For this review, take the finished solid that the model builds, in its own axes (mm). Face numbers are marked on the shaded views. A direction names the side the tool comes from. Give positions to 0.01 mm unless a question says otherwise; leave off trailing zeros. Order: outer loops, then holes, each group sorted by start corner. A loop starts at its lowest first (then second) coordinate and runs counter-clockwise, first axis right, second up. Notation, with made-up numbers: (-7.75, 21.5) -> (47.25, 21.5) arc R27 ccw to (47.25, 42.5) -> close; hole circle Ø5 at (27, 38.5). An arc over 180 degrees is marked (long way). One line per item, written item: value. Start each with the question number.
from build123d import *

# Parameters (mm, degrees)
PAD_DEPTH        = 8
SKETCH001_W      = 60
SKETCH001_H      = 5
PAD001_DEPTH     = 240
POCKET_DEPTH     = 5.001
POCKET001_DEPTH  = 5.001
PAD002_DEPTH     = 8
HOLE_D           = 4.4
HOLE_CSINK_D     = 8
HOLE_CSINK_ANGLE = 90


with BuildPart() as part:
    # Sketch → Pad (new body)
    with BuildSketch(Plane.XZ):
        with BuildLine():
            Line((-30, 0), (30, 0))
            Line((30, 0), (30, -30))
            Line((30, -30), (20.25, -30))
            Line((20.25, -22.145781), (20.25, -30))
            ThreePointArc((20.25, -22.145781), (14, -10.5), (7.75, -22.145781))
            Line((7.75, -22.145781), (7.75, -30))
            Line((7.75, -30), (-7.75, -30))
            Line((-7.75, -22.145781), (-7.75, -30))
            ThreePointArc((-7.75, -22.145781), (-14, -10.5), (-20.25, -22.145781))
            Line((-20.25, -22.145781), (-20.25, -30))
            Line((-20.25, -30), (-30, -30))
            Line((-30, -30), (-30, 0))
        make_face()
    extrude(amount=PAD_DEPTH)

    # Sketch001 (on Face14 of Pad) → Pad001 (join)
    with BuildSketch(Plane.XZ.offset(8)):
        with Locations((0, -2.5)):
            Rectangle(SKETCH001_W, SKETCH001_H)
    extrude(amount=PAD001_DEPTH)

    # Sketch002 (on Face15 of Pad001) → Pocket (cut, through all)
    with BuildSketch(Plane(origin=(0, 0, -5), x_dir=(1, 0, 0), z_dir=(0, 0, -1))):
        Polygon((-19.5, 251), (-33, 251), (-33, 0.857143), (-19.5, 33), align=None)
    extrude(amount=-POCKET_DEPTH, mode=Mode.SUBTRACT)

    # Sketch003 (on Face15 of Pocket) → Pocket001 (cut, through all)
    with BuildSketch(Plane(origin=(0, 0, -5), x_dir=(1, 0, 0), z_dir=(0, 0, -1))):
        Polygon((19.5, 251), (33, 251), (33, 0.857143), (19.5, 33), align=None)
    extrude(amount=-POCKET001_DEPTH, mode=Mode.SUBTRACT)

    # Sketch004 (on Face20 of Pocket001) → Pad002 (join)
    with BuildSketch(Plane.XZ.offset(248)):
        with BuildLine():
            Line((-19.5, 0), (19.5, 0))
            Line((19.5, 0), (19.5, -30))
            Line((19.5, -30), (18, -30))
            Line((18, -27), (18, -30))
            ThreePointArc((18, -27), (14, -20.438447), (10, -27))
            Line((10, -27), (10, -30))
            Line((10, -30), (-10, -30))
            Line((-10, -27), (-10, -30))
            ThreePointArc((-10, -27), (-14, -20.438447), (-18, -27))
            Line((-18, -27), (-18, -30))
            Line((-18, -30), (-19.5, -30))
            Line((-19.5, -30), (-19.5, 0))
        make_face()
    extrude(amount=-PAD002_DEPTH)

    # Hole (through all)
    with Locations(Plane(origin=(0, 0, -5), x_dir=(1, 0, 0), z_dir=(0, 0, -1))):
        with Locations((0, 30), (0, 130)):
            CounterSinkHole(HOLE_D / 2, HOLE_CSINK_D / 2, counter_sink_angle=HOLE_CSINK_ANGLE)


solid = part.part
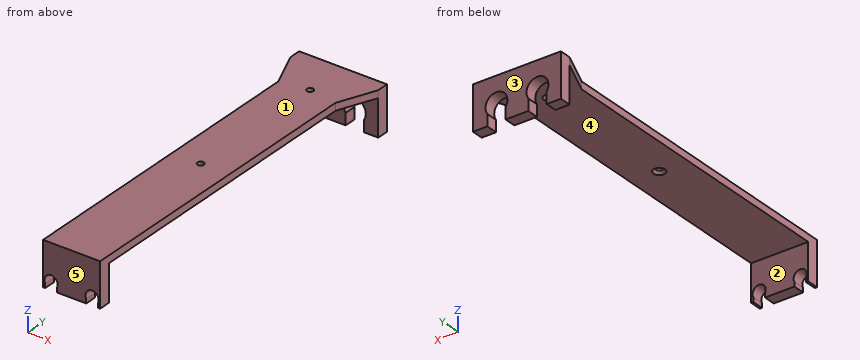
Q1. For pin 1 Ø8 at (x, y) = (10, -223) entering from +Z; pin 2 Ø12 at (y, z) = (-136, -7) entering from -X; pin 3 Ø8 at (x, y) = (12.5, -208.5) entering from -Z; pin 4 Ø2.5 at (y, z) = (-243, -28) entering from +X, all flat-tipped, find the tip position at first contact; note any pin that passes through.
Q2. Take a section at D-D (x = 14). State the section outline as (y, z) points, and give its area (3 significant figures).
Q3. Take a section at C-C (z = -18). State the section outline as (x, y) points, and give its area (3 significant figures).
Q4. For the marked faces 4 and 5, list the 3-axis set-ups (+Z, -Z, +X, -X, +Y, -Y) from which the entire face can be reached by the end or side of a thin tool; tool diameter is ignored.
Q5. Mouldability with a two-part tool opening along Y and no side actions: class the marked faces 1, 2 and 3 as pulls with the +Y half, pulls with the -Y half, needs draft (parallel to the pull), parting line crosses it, or undercut.
Q6. Take a section at A-A (y = -30). State the section outline as (x, z) points, and give its area (3 significant figures).
Q7. For line 1 along X through (y, z) = (-6.25, -18); line 2 along Y through (x, z) = (0, -2.4); line 3 along X through (y, z) = (-130, -2.2), list the stretches that pass through material, from the lowest coordinate up.
Q8. Take a section at B-B (x = 0). State the section outline as (y, z) points.
Answers below:
1. pin 1: stops at z = 0
1. pin 2: stops at x = -19.5
1. pin 3: stops at z = -5
1. pin 4: stops at x = 19.5
2. outline: (-248, -20.44) -> (-240, -20.44) -> (-240, -5) -> (-8, -5) -> (-8, -10.5) -> (0, -10.5) -> (0, 0) -> (-248, 0) -> close
2. area: 1,410 mm²
3. outline: (-30, -8) -> (-21.5, -8) -> (-21.5, 0) -> (-30, 0) -> close; (-19.5, -248) -> (19.5, -248) -> (19.5, -240) -> (-19.5, -240) -> close; (-6.5, -8) -> (6.5, -8) -> (6.5, 0) -> (-6.5, 0) -> close; (21.5, -8) -> (30, -8) -> (30, 0) -> (21.5, 0) -> close
3. area: 552 mm²
4. face 4: -Z, +X, -X
4. face 5: +Z, -Z, +X, -X, -Y
5. face 1: needs draft
5. face 2: undercut
5. face 3: pulls with the +Y half
6. outline: (-20.76, -5) -> (-4, -5) -> (-2.2, -3.2) -> (-2.2, 0) -> (-20.76, 0) -> close; (2.2, -3.2) -> (4, -5) -> (20.76, -5) -> (20.76, 0) -> (2.2, 0) -> close
6. area: 182 mm²
7. line 1: x = -30 to -21.5, -6.5 to 6.5, 21.5 to 30
7. line 2: y = -248 to -132.2, -127.8 to -32.2, -27.8 to 0
7. line 3: x = -19.5 to -2.2, 2.2 to 19.5
8. outline: (-248, -30) -> (-240, -30) -> (-240, -5) -> (-134, -5) -> (-132.2, -3.2) -> (-132.2, 0) -> (-248, 0) -> close; (-127.8, -3.2) -> (-126, -5) -> (-34, -5) -> (-32.2, -3.2) -> (-32.2, 0) -> (-127.8, 0) -> close; (-27.8, -3.2) -> (-26, -5) -> (-8, -5) -> (-8, -30) -> (0, -30) -> (0, 0) -> (-27.8, 0) -> close
